Work out the finished part from the listing and answer in its coordinate system (mm). Round coordinates to 2 decimals unless told otherwise and drop trailing zeros. Write each loop counter-clockwise with the first axis right and the second up, starting at its lowest first coordinate (ties: lowest second). Pieces come first, ordered by that corner, then holes. Notation, with made-up numbers: M 3,77.5 L 53,77.5 A25 cw 53,103.5 Z; hole C -34.5,82.25 d4. An arc over 180 degrees is marked long. Answer in a Markdown table with one row per item.
```python
from build123d import *

# Parameters (mm, degrees)
SALIENTE_EXTRUIR1_DEPTH = 25.4


with BuildPart() as part:
    # Croquis2 → Saliente-Extruir1 (new body)
    with BuildSketch(Plane(origin=(0, 0, 0), x_dir=(1, 0, 0), z_dir=(0, 1, 0))):
        Polygon((0, 0), (101.6, 0), (101.6, 19.443856069), (63.5, 46.121763275), (0, 34.925), align=None)
    extrude(amount=SALIENTE_EXTRUIR1_DEPTH)


solid = part.part
```
1. The part is cut by section B-B (z = -39). Determine the outline of the cut face in (x, y).
Calculated:
| item | result |
|---|---|
| outline | M 23.11,0 L 73.67,0 L 73.67,25.4 L 23.11,25.4 Z |
2. The part is cut by section A-A (y = 2.25). Determine the outline of the cut face in (x, z) (3 decimals), plus the area to 3 significant figures.
Calculated:
| item | result |
|---|---|
| outline | M 0,-34.925 L 63.5,-46.122 L 101.6,-19.444 L 101.6,0 L 0,0 Z |
| area | 3,820 mm² |
3. Consider line 1 along Z through (x, y) = (57, 21); line 2 along Z through (x, y) = (22, 20.5); line 3 along X through (y, z) = (22.75, -26). Determine where each line is inside the solid, lowest interval first. Write a range as from..to.
Calculated:
| item | result |
|---|---|
| line 1 | z = -44.98..0 |
| line 2 | z = -38.8..0 |
| line 3 | x = 0..92.24 |
4. The part is cut by section C-C (x = 53). Determine the outline of the cut face in (y, z), plus the area to 3 significant figures.
Calculated:
| item | result |
|---|---|
| outline | M 0,-44.27 L 25.4,-44.27 L 25.4,0 L 0,0 Z |
| area | 1,120 mm² |
